from build123d import *

# Parameters (mm, degrees)
F0_W     = 139.7
F0_H     = 139.7
F1_DEPTH = 6.35
F2_W     = 6.35
F2_H     = 6.35
F2_W_2   = 18.1428571429
F2_H_2   = 18.1428571429
F3_DEPTH = 25.4


with BuildPart() as f1:
    # F0 (on Front) → F1 (new body)
    with BuildSketch(Plane.XZ):
        Rectangle(F0_W, F0_H)
    extrude(amount=F1_DEPTH)

    # F2 (on face) → F3 (cut)
    with BuildSketch(Plane.XZ.offset(6.35)):
        with Locations((-66.675, 66.675)):
            Rectangle(F2_W, F2_H)
        with Locations((-36.2857142857, 66.675)):
            Rectangle(F2_W_2, F2_H)
        with Locations((0, 66.675)):
            Rectangle(F2_W_2, F2_H)
        with Locations((36.2857142857, 66.675)):
            Rectangle(F2_W_2, F2_H)
        with Locations((66.675, 66.675)):
            Rectangle(F2_W, F2_H)
        with Locations((66.675, 36.2857142857)):
            Rectangle(F2_W, F2_H_2)
        with Locations((66.675, 0)):
            Rectangle(F2_W, F2_H_2)
        with Locations((66.675, -36.2857142857)):
            Rectangle(F2_W, F2_H_2)
        with Locations((66.675, -66.675)):
            Rectangle(F2_W, F2_H)
        with Locations((36.2857142857, -66.675)):
            Rectangle(F2_W_2, F2_H)
        with Locations((0, -66.675)):
            Rectangle(F2_W_2, F2_H)
        with Locations((-36.2857142857, -66.675)):
            Rectangle(F2_W_2, F2_H)
        with Locations((-66.675, -66.675)):
            Rectangle(F2_W, F2_H)
        with Locations((-66.675, -36.2857142857)):
            Rectangle(F2_W, F2_H_2)
        with Locations((-66.675, 0)):
            Rectangle(F2_W, F2_H_2)
        with Locations((-66.675, 36.2857142857)):
            Rectangle(F2_W, F2_H_2)
    extrude(amount=-F3_DEPTH, mode=Mode.SUBTRACT)


solid = f1.part
Design review of the part built by this model. Coordinates are the model's own, in mm. A direction names the side the tool comes from. Give positions to 0.01 mm unless a question says otherwise; leave off trailing zeros. Loops run counter-clockwise (first coordinate to the right, second up) from the corner with the lowest first, then second, coordinate; pieces in that order, holes last. Notation, with made-up numbers: (9, -21) - (28, -21) arc R23 cw to (28, 0) - close; hole circle Ø9 at (61.25, 31.25). An arc over 180 degrees is marked (long way). Write item = value, one per line.
1) Take a section at B-B on z = -32. State the section outline as (x, y) points, and give its area (3 significant figures).
Result sheet:
outline = (-63.5, -6.35) - (63.5, -6.35) - (63.5, 0) - (-63.5, 0) - close
area = 806 mm2
2) Clearance check with flat-ended pins moving along their axes: pin 1 Ø1.5 at (x, y) = (-41.5, -4) entering from -Z; pin 2 Ø3 at (y, z) = (-4, 68) entering from -X; pin 3 Ø1.9 at (x, y) = (-68, -3) entering from +Z. State where each tip first meets the part, or that it passes through.
Result sheet:
pin_1 = -63.5
pin_2 = -63.5
pin_3 = 63.5
3) Tool access review of faces 1 (the face through (-67, -3, 63.5)), 2 (the face through (-67, -3, -45.357)), 3 (the face through (63.5, -3, 36)): name each direction out of +Z, -Z, +X, -X, +Y, -Y from which nothing blocks a thin tool from reaching the whole face with its end or side.
Result sheet:
face_1 = +Z, -X, +Y, -Y
face_2 = -X, +Y, -Y
face_3 = +X, +Y, -Y
4) Draft analysis for pull direction X (two halves, no side actions). For faces 4 (the face through (-63.5, -3, 0)), 5 (the face through (-27.214, -3, 67)), 6 (the face through (67, -3, -9.071)), 7 (the face through (36, -3, -63.5)), state which applies: +X half, -X half, draft (parallel to the pull), parting line (faces both ways), or undercut.
Result sheet:
face_4 = -X half
face_5 = undercut
face_6 = draft
face_7 = undercut
5) To check wall thickness, follow line 1 (Z direction, x = 64, y = -3); line 2 (X direction, y = -2.25, z = 35). State the ranges of each line that lie inside material, in increasing order.
Result sheet:
line_1 = -63.5 to -45.36, -27.21 to -9.07, 9.07 to 27.21, 45.36 to 63.5
line_2 = -63.5 to 63.5
6) Take a section at A-A on x = 41. State the section outline as (y, z) points.
Result sheet:
outline = (-6.35, -63.5) - (0, -63.5) - (0, 63.5) - (-6.35, 63.5) - close
